Input: part model. Units: mm. Frame: model coordinates. A direction names the side the tool comes from. Coordinates: 2 decimals unless noted, no trailing zeros. Write each loop counter-clockwise with the first axis right and the second up, starting at its lowest first coordinate (ties: lowest second). Pieces come first, ordered by that corner, then holes. Notation, with made-up numbers: M 34.25,31 L 39.25,31 A5 ccw 39.25,39 Z; hole C 56.5,-5.5 d4. An arc over 180 degrees is marked long. Use one line per item in the form item = value.
from build123d import *

# Parameters (mm, degrees)
SKETCH1_W           = 15
SKETCH1_H           = 20
BOSS_EXTRUDE1_DEPTH = 6
SKETCH2_W           = 10
SKETCH2_H           = 3
CUT_EXTRUDE1_DEPTH  = 16
FILLET1_R           = 5
FILLET2_R           = 5
FILLET3_R           = 2
SKETCH3_R           = 1
CUT_EXTRUDE2_DEPTH  = 16


with BuildPart() as part:
    # Sketch1 → Boss-Extrude1 (new body)
    with BuildSketch(Plane(origin=(0, 0, 0), x_dir=(1, 0, 0), z_dir=(0, 1, 0))):
        Rectangle(SKETCH1_W, SKETCH1_H)
    extrude(amount=BOSS_EXTRUDE1_DEPTH)

    # Sketch2 → Cut-Extrude1 (cut)
    with BuildSketch(Plane.XY.offset(10)):
        with Locations((0, 3)):
            Rectangle(SKETCH2_W, SKETCH2_H)
    extrude(amount=-CUT_EXTRUDE1_DEPTH, mode=Mode.SUBTRACT)

    # Fillet1
    fillet1_edges = [part.edges().sort_by_distance(p)[0] for p in [
        (7.5, 3, -10),
    ]]
    fillet(fillet1_edges, radius=FILLET1_R)

    # Fillet2
    fillet2_edges = [part.edges().sort_by_distance(p)[0] for p in [
        (-7.5, 3, -10),
    ]]
    fillet(fillet2_edges, radius=FILLET2_R)

    # Fillet3
    fillet3_edges = [part.edges().sort_by_distance(p)[0] for p in [
        (7.5, 6, 2.5),
        (0, 0, -10),
        (0, 6, -10),
        (6.035533906, 0, -8.535533906),
        (6.035533906, 6, -8.535533906),
        (-7.5, 0, 2.5),
        (-7.5, 6, 2.5),
        (-6.035533906, 0, -8.535533906),
        (-6.035533906, 6, -8.535533906),
        (7.5, 0, 2.5),
    ]]
    fillet(fillet3_edges, radius=FILLET3_R)

    # Sketch3 → Cut-Extrude2 (cut)
    with BuildSketch(Plane.XZ):
        with Locations(Location((0, 0, 0), (0, 0, 270))):
            Circle(SKETCH3_R)
    extrude(amount=-CUT_EXTRUDE2_DEPTH, mode=Mode.SUBTRACT)


solid = part.part
(1) Section query B-B on y = 3.3. Return the cut outline in (x, z), plus the area to 3 significant figures.
Computed:
outline = M -7.5,-5 A5 ccw -2.5,-10 L 2.5,-10 A5 ccw 7.5,-5 L 7.5,10 L 5,10 L 5,-6 L -5,-6 L -5,10 L -7.5,10 Z
area = 129 mm^2
(2) Pull-direction query (Y, two-part tool) for faces 3 (the cylindrical face through (6.93, 0.6, 2.61)), 4 (the flat face through (0, 4.5, 2)), 5 (the cylindrical face through (-1, 5, 0)); classes: pulls with the +Y half, pulls with the -Y half, needs draft (parallel to the pull), parting line crosses it, or undercut.
Computed:
face_3 = pulls with the -Y half
face_4 = undercut
face_5 = needs draft
(3) Set-up query: faces 1 (the cylindrical face through (-1, 1, 0)), 2 (the flat face through (5, 3, 2)). Return all of +Z, -Z, +X, -X, +Y, -Y with unobstructed straight access to the full face (end or side cutting, diameter ignored); none if empty.
Computed:
face_1 = +Y, -Y
face_2 = +Z
(4) Section query D-D on z = 8. Return the cut outline in (x, y), plus the area to 3 significant figures.
Computed:
outline = M -7.5,2 A2 ccw -5.5,0 L 5.5,0 A2 ccw 7.5,2 L 7.5,4 A2 ccw 5.5,6 L -5.5,6 A2 ccw -7.5,4 Z; hole M -5,1.5 L 5,1.5 L 5,4.5 L -5,4.5 Z
area = 56.6 mm^2
(5) First-contact query: pin 1 Ø1.5 at (x, y) = (-2.5, 2.5) entering from +Z. Flat tip, straight axial feed; report the tip coordinate or a pass-through.
Computed:
pin_1 = -6
(6) Section query C-C on x = 0. Return the cut outline in (y, z), plus the area to 3 significant figures.
Computed:
outline = M 0,-8 A2 ccw 2,-10 L 4,-10 A2 ccw 6,-8 L 6,-1 L 4.5,-1 L 4.5,-6 L 1.5,-6 L 1.5,-1 L 0,-1 Z; M 0,1 L 1.5,1 L 1.5,10 L 0,10 Z; M 4.5,1 L 6,1 L 6,10 L 4.5,10 Z
area = 64.3 mm^2
(7) Line query: probe 1 along Y at (x, z) = (2.25, 6); probe 2 along X at (y, z) = (3.95, 4.25); probe 3 along Z at (x, y) = (-2, 2.2). Output: solid intervals per line, ascending.
Computed:
probe_1 = 0 to 1.5, 4.5 to 6
probe_2 = -7.5 to -5, 5 to 7.5
probe_3 = -10 to -6
(8) Section query A-A on z = 0. Return the cut outline in (x, y).
Computed:
outline = M -7.5,2 A2 ccw -5.5,0 L -1,0 L -1,1.5 L -5,1.5 L -5,4.5 L -1,4.5 L -1,6 L -5.5,6 A2 ccw -7.5,4 Z; M 1,0 L 5.5,0 A2 ccw 7.5,2 L 7.5,4 A2 ccw 5.5,6 L 1,6 L 1,4.5 L 5,4.5 L 5,1.5 L 1,1.5 Z
